Geometry: final body of the model. Coordinates: model frame, mm. Give positions to 0.01 mm unless a question says otherwise; leave off trailing zeros. Write each loop counter-clockwise with the first axis right and the second up, starting at its lowest first coordinate (ties: lowest second). Pieces come first, ordered by that corner, then holes. Notation, with made-up numbers: M -24.75,-24 L 26.25,-24 A14 ccw 26.25,2 Z; hole C 46,-15.75 d8. An arc over 180 degrees is marked long. Use a Markdown table: item, result. Add a question column.
(1) Draft query along X for faces 1 (the flat face through (20, 89, 3)), 2 (the flat face through (-71, 0, 3)), 3 (the cylindrical face through (-120.782, 61.263, 2.958)). Return one class per face: released by +X, released by -X, zero draft, split by the parting line, or undercut.
(2) Cut plane C-C (x = -58.52). Output: boundary loops of the cut face in (y, z).
(3) Cut plane D-D (y = 112). Output: boundary loops of the cut face in (x, z).
(4) Pin query (flat end, axial travel): pin 1 Ø8 at (x, y) = (-58.52, 17.52) entering from +Z; pin 2 Ø2.5 at (y, z) = (100.5, 5) entering from -X; pin 3 Ø1 at (y, z) = (78, 5) entering from -X; pin 4 Ø1.5 at (x, z) = (14, 4.5) entering from -Y (3 decimals). Return the tip coordinate at first contact, or that it passes through.
(5) Material intervals for L1, parallel to X at y = 17.52, z = 3.75 (3 decimals); L2, parallel to Z at x = 2, y = 90; L3, parallel to X at y = 110, z = 3.6, sorted ascending.
(6) Cut plane A-A (y = 17.52). Output: boundary loops of the cut face in (x, z) (3 decimals), plus the area to 3 significant figures.
(7) Cut plane B-B (z = 5.1). Output: boundary loops of the cut face in (x, y) (1 decimal).
Solid Edge part; units mm, degrees
sketch "Sketch1" plane through (0, 0, 0) normal (0, 0, 1) x (1, 0, 0)
  line L0 (0, 0) -> (-165.365, 0)
  line L1 (-165.365, 0) -> (-165.365, 50)
  arc A0 (-165.365, 50) -> (-34.465, 180.07) centre (-35.291, 49.9987) cw
  line L2 (0, 180.07) -> (-34.465, 180.07)
  line L3 (0, 0) -> (0, 180.07)
  circle A1 centre (-47.0756, 132.1051) radius 2.9988
  circle A2 centre (-117.7863, 61.3945) radius 2.9988
  dimension "D1" = 165.365
extrude "Protrusion1" add sketch "Sketch1" along normal blind 6
sketch "Sketch2" plane through (0, 90.035, 3) normal (1, 0, 0) x (0, 1, 0)
  line L0 (-90.035, 3) -> (90.035, 3)
  line L1 (90.035, 3) -> (90.035, -3)
  line L2 (90.035, -3) -> (-90.035, -3)
  line L3 (-90.035, -3) -> (-90.035, 3)
extrude "Extrusionsausprägung_2" add sketch "Sketch2" along normal blind 20
sketch "Sketch3" plane through (-72.6825, 90.0363, 6) normal (0, 0, 1) x (1, 0, 0)
  line L0 (92.6825, 90.0337) -> (72.6825, 90.0337)
  line L1 (72.6825, 90.0337) -> (72.6825, -90.0363)
  line L2 (72.6825, -90.0363) -> (92.6825, -90.0363)
  line L3 (92.6825, -90.0363) -> (92.6825, -70.0013)
  line L4 (82.6825, -70.0013) -> (92.6825, -70.0013)
  line L5 (82.6825, 69.9987) -> (82.6825, -70.0013)
  line L6 (92.6825, 69.9987) -> (82.6825, 69.9987)
  line L7 (92.6825, 90.0337) -> (92.6825, 69.9987)
extrude "Extrusionsausschnitt_1" cut sketch "Sketch3" against normal blind 3
sketch "Sketch4" plane through (-72.6825, 90.0363, 0) normal (0, 0, -1) x (0, 1, 0)
  circle A0 centre (-72.5163, 54.1625) radius 3.5
  circle A1 centre (-72.5163, 14.1625) radius 3.5
  dimension "D1" = 72.5163
extrude "Cutout1" cut sketch "Sketch4" against normal through all
properties material "Nylon, allgemein"
Answer list:
| question | item | result |
|---|---|---|
| 1 | face 1 | released by +X |
| 1 | face 2 | zero draft |
| 1 | face 3 | undercut |
| 2 | outline | M 0,0 L 14.02,0 L 14.02,6 L 0,6 Z; M 21.02,0 L 177.98,0 L 177.98,6 L 21.02,6 Z |
| 3 | outline | M -149.64,0 L 20,0 L 20,6 L 10,6 L 10,3 L 0,3 L 0,6 L -149.64,6 Z |
| 4 | pin 1 | z = 6 |
| 4 | pin 2 | x = -155.68 |
| 4 | pin 3 | x = -162.42 |
| 4 | pin 4 | y = 20.035 |
| 5 | L1 | -165.365 to -62.02, -55.02 to -22.02, -15.02 to 0 |
| 5 | L2 | 0 to 3 |
| 5 | L3 | -150.7 to 0, 10 to 20 |
| 6 | outline | M -165.365,0 L -62.02,0 L -62.02,6 L -165.365,6 Z; M -55.02,0 L -22.02,0 L -22.02,6 L -55.02,6 Z; M -15.02,0 L 20,0 L 20,3 L 0,3 L 0,6 L -15.02,6 Z |
| 6 | area | 968 mm² |
| 7 | outline | M -165.4,0 L 0,0 L 0,180.1 L -34.5,180.1 A130.1 ccw -165.4,50 Z; M 10,20 L 20,20 L 20,160 L 10,160 Z; hole C -117.8,61.4 d6; hole C -58.5,17.5 d7; hole C -47.1,132.1 d6; hole C -18.5,17.5 d7 |
